Source: CAD feature listing. Evaluate the final solid. Frame: model axes, mm. A direction names the side the tool comes from. Give positions to 0.01 mm unless a question says otherwise; leave off trailing zeros. Write each loop counter-clockwise with the first axis right and the second up, starting at its lowest first coordinate (ties: lowest second). Pieces come first, ordered by that corner, then holes. Notation, with made-up numbers: M 18,-21.5 L 35,-21.5 A31 cw 35,12.5 Z; hole C -3.5,-2 d2. An arc over 180 degrees is marked long. Return JSON: item names as keys, results as strings.
```python
from build123d import *

# Parameters (mm, degrees)
SKETCH_1_W          = 108
SKETCH_1_H          = 138
EXTRUDE_1_DEPTH     = 4
SKETCH_2_W          = 69.21
SKETCH_2_H          = 50.1
CUT_EXTRUDE_1_DEPTH = 176.282628917
SKETCH_3_W          = 12.1
SKETCH_3_H          = 12.1
SKETCH_3_H_2        = 12.45
SKETCH_3_W_2        = 12.45
CUT_EXTRUDE_2_DEPTH = 176.282628917
SKETCH_4_W          = 15
SKETCH_4_H          = 4
EXTRUDE_2_DEPTH     = 6
SKETCH_6_W          = 9
SKETCH_6_H          = 4
EXTRUDE_3_DEPTH     = 6
SKETCH_7_W          = 15
SKETCH_7_H          = 4
EXTRUDE_4_DEPTH     = 6
SKETCH_8_W          = 9
SKETCH_8_H          = 4
EXTRUDE_5_DEPTH     = 6
SKETCH_9_W          = 10
SKETCH_9_H          = 4
EXTRUDE_6_DEPTH     = 6


with BuildPart() as part:
    # Эскиз1 → Бобышка-Вытянуть1 (new body)
    with BuildSketch(Plane(origin=(0, 0, 0), x_dir=(1, 0, 0), z_dir=(0, 1, 0))):
        with Locations((54, -69)):
            Rectangle(SKETCH_1_W, SKETCH_1_H)
    extrude(amount=EXTRUDE_1_DEPTH)

    # Эскиз2 → Вырез-Вытянуть1 (cut, through all)
    with BuildSketch(Plane(origin=(0, 4, 0), x_dir=(1, 0, 0), z_dir=(0, 1, 0))):
        with Locations((48.205, -35.05)):
            Rectangle(SKETCH_2_W, SKETCH_2_H)
    extrude(amount=-CUT_EXTRUDE_1_DEPTH, mode=Mode.SUBTRACT)

    # Эскиз3 → Вырез-Вытянуть2 (cut, through all)
    with BuildSketch(Plane(origin=(0, 4, 0), x_dir=(1, 0, 0), z_dir=(0, 1, 0))):
        with Locations((24.022320969, -115.030109588)):
            Rectangle(SKETCH_3_W, SKETCH_3_H)
        with Locations((24.022320969, -102.755109588)):
            Rectangle(SKETCH_3_W, SKETCH_3_H_2)
        with Locations((11.747320969, -115.030109588)):
            Rectangle(SKETCH_3_W_2, SKETCH_3_H)
        with Locations((36.297320969, -115.030109588)):
            Rectangle(SKETCH_3_W_2, SKETCH_3_H)
        with Locations((24.022320969, -127.305109588)):
            Rectangle(SKETCH_3_W, SKETCH_3_H_2)
    extrude(amount=-CUT_EXTRUDE_2_DEPTH, mode=Mode.SUBTRACT)

    # Эскиз4 → Бобышка-Вытянуть2 (add)
    with BuildSketch(Plane.ZY):
        with Locations((11.5, 2)):
            Rectangle(SKETCH_4_W, SKETCH_4_H)
        with Locations((36.5, 2)):
            Rectangle(SKETCH_4_W, SKETCH_4_H)
        with Locations((61.5, 2)):
            Rectangle(SKETCH_4_W, SKETCH_4_H)
        with Locations((86.5, 2)):
            Rectangle(SKETCH_4_W, SKETCH_4_H)
        with Locations((111.5, 2)):
            Rectangle(SKETCH_4_W, SKETCH_4_H)
    extrude(amount=EXTRUDE_2_DEPTH)

    # Эскиз6 → Бобышка-Вытянуть3 (add)
    with BuildSketch(Plane.ZY):
        with Locations((133.5, 2)):
            Rectangle(SKETCH_6_W, SKETCH_6_H)
    extrude(amount=EXTRUDE_3_DEPTH)

    # Эскиз7 → Бобышка-Вытянуть4 (add)
    with BuildSketch(Plane(origin=(108, 0, 0), x_dir=(0, 0, -1), z_dir=(1, 0, 0))):
        with Locations((-11.5, 2)):
            Rectangle(SKETCH_7_W, SKETCH_7_H)
        with Locations((-36.5, 2)):
            Rectangle(SKETCH_7_W, SKETCH_7_H)
        with Locations((-61.5, 2)):
            Rectangle(SKETCH_7_W, SKETCH_7_H)
        with Locations((-86.5, 2)):
            Rectangle(SKETCH_7_W, SKETCH_7_H)
        with Locations((-111.5, 2)):
            Rectangle(SKETCH_7_W, SKETCH_7_H)
    extrude(amount=EXTRUDE_4_DEPTH)

    # Эскиз8 → Бобышка-Вытянуть5 (add)
    with BuildSketch(Plane(origin=(108, 0, 0), x_dir=(0, 0, -1), z_dir=(1, 0, 0))):
        with Locations((-133.5, 2)):
            Rectangle(SKETCH_8_W, SKETCH_8_H)
    extrude(amount=EXTRUDE_5_DEPTH)

    # Эскиз9 → Бобышка-Вытянуть6 (add)
    with BuildSketch(Plane(origin=(0, 0, 0), x_dir=(-1, 0, 0), z_dir=(0, 0, -1))):
        with Locations((-94.998495411, 2)):
            Rectangle(SKETCH_9_W, SKETCH_9_H)
        with Locations((-74.998495411, 2)):
            Rectangle(SKETCH_9_W, SKETCH_9_H)
        with Locations((-54.998495411, 2)):
            Rectangle(SKETCH_9_W, SKETCH_9_H)
        with Locations((-34.998495411, 2)):
            Rectangle(SKETCH_9_W, SKETCH_9_H)
        with Locations((-14.998495411, 2)):
            Rectangle(SKETCH_9_W, SKETCH_9_H)
    extrude(amount=EXTRUDE_6_DEPTH)


solid = part.part
```
1) Cut plane C-C, the plane x = 27. Return the cut outline in (y, z), then the cut area to 3 significant figures.
Numbers:
{"outline": "M 0,0 L 4,0 L 4,10 L 0,10 Z; M 0,60.1 L 4,60.1 L 4,96.53 L 0,96.53 Z; M 0,133.53 L 4,133.53 L 4,138 L 0,138 Z", "area": "204 mm²"}
2) Draft query along Z for faces 6 (the face through (75, 2, -6)), 7 (the face through (111, 2, 119)), 8 (the face through (53, 0, 67)). Return one class per face: released by +Z, released by -Z, zero draft, split by the parting line, or undercut.
Numbers:
{"face 6": "released by -Z", "face 7": "undercut", "face 8": "zero draft"}
3) Set-up query: faces 1 (the face through (49.998, 2, -3)), 2 (the face through (0, 2, 2)), 3 (the face through (111, 2, 54)), 4 (the face through (48, 2, 10)), 5 (the face through (0, 2, 99)). Return all of +Z, -Z, +X, -X, +Y, -Y with unobstructed straight access to the full face (end or side cutting, diameter ignored); none if empty.
Numbers:
{"face 1": "-Z, +Y, -Y", "face 2": "-Z, -X, +Y, -Y", "face 3": "+X, +Y, -Y", "face 4": "+Y, -Y", "face 5": "-X, +Y, -Y"}
4) Line query: line 1 (Z direction, x = 23.5, y = 2.35); line 2 (Z direction, x = 58, y = 3.05); line 3 (Z direction, x = 49, y = 0.9). Output: solid intervals per line, ascending. Write a range as [from, to].
Numbers:
{"line 1": "z = [0, 10], [60.1, 96.53], [133.53, 138]", "line 2": "z = [-6, 10], [60.1, 138]", "line 3": "z = [0, 10], [60.1, 138]"}
5) Cut plane A-A, the plane z = 42. Return the cut outline in (x, y), then the cut area to 3 significant figures.
Numbers:
{"outline": "M -6,0 L 13.6,0 L 13.6,4 L -6,4 Z; M 82.81,0 L 114,0 L 114,4 L 82.81,4 Z", "area": "203 mm²"}
6) Cut plane B-B, the plane x = 7.5. Return the cut outline in (y, z), then the cut area to 3 significant figures.
Numbers:
{"outline": "M 0,0 L 4,0 L 4,108.98 L 0,108.98 Z; M 0,121.08 L 4,121.08 L 4,138 L 0,138 Z", "area": "504 mm²"}
7) Contact query for flat-ended pins moving along their axis: pin 1 Ø1.2 at (y, z) = (2, 100) entering from +X; pin 2 Ø2 at (x, y) = (27, 3) entering from -Z; pin 3 Ø1.2 at (y, z) = (1.5, -1.5) entering from -X. Output: stop coordinate, or through.
Numbers:
{"pin 1": "stops at x = 108", "pin 2": "stops at z = 0", "pin 3": "stops at x = 10"}
8) Cut plane D-D, the plane y = 2.25. Give the number of separate pieces and of enclosed holes in the cut face, then the cut area to 3 significant figures.
Numbers:
{"separate pieces": "1", "enclosed holes": "2", "area": "12,000 mm²"}
